from build123d import *

# Parameters (mm, degrees)
BOSS_EXTRUDE1_START = 20
BOSS_EXTRUDE1_DEPTH = 20
CIRPATTERN1_COUNT   = 9


with BuildPart() as part:
    # Sketch1 → Revolve1 (revolve)
    with BuildSketch(Plane.XY):
        Polygon((-50, 0), (-50, 100), (0, 100), (0, 420), (-30, 420), (-30, 465), (-10, 465), (10.490381057, 459.509618943), (30, 440), (30, 0), align=None)
    revolve(axis=Axis((30, 0, 0), (-1, 0, 0)))

    # Sketch2 → Boss-Extrude1 (add)
    with BuildSketch(Plane.ZY.offset(BOSS_EXTRUDE1_START)):
        with BuildLine():
            ThreePointArc((27.272727273, 96.209138584), (22.022759648, 99.799825551), (20, 105.830052443))
            Line((20, 105.830052443), (20, 408.900966005))
            ThreePointArc((20, 408.900966005), (23.192543543, 416.226164746), (30.731707317, 418.874160298))
            ThreePointArc((30.731707317, 418.874160298), (5.43490171, 419.964834056), (-19.881656805, 419.529164329))
            ThreePointArc((-19.881656805, 419.529164329), (-56.82924306, 416.1375219), (-93.333333333, 409.498338078))
            ThreePointArc((-93.333333333, 409.498338078), (-42.583426132, 397.902733094), (-20, 350.998575496))
            Line((-20, 350.998575496), (-20, 105.830052443))
            ThreePointArc((-20, 105.830052443), (-22.022759648, 99.799825551), (-27.272727273, 96.209138584))
            ThreePointArc((-27.272727273, 96.209138584), (0, 100), (27.272727273, 96.209138584))
        make_face()
    boss_extrude1 = extrude(amount=-BOSS_EXTRUDE1_DEPTH)

    # CirPattern1: Boss-Extrude1 ×9 about axis
    cirpattern1_axis = Axis((0, 0, 0), (1, 0, 0))
    for i in range(1, CIRPATTERN1_COUNT):
        add(boss_extrude1.rotate(cirpattern1_axis, i * 360 / CIRPATTERN1_COUNT))


solid = part.part
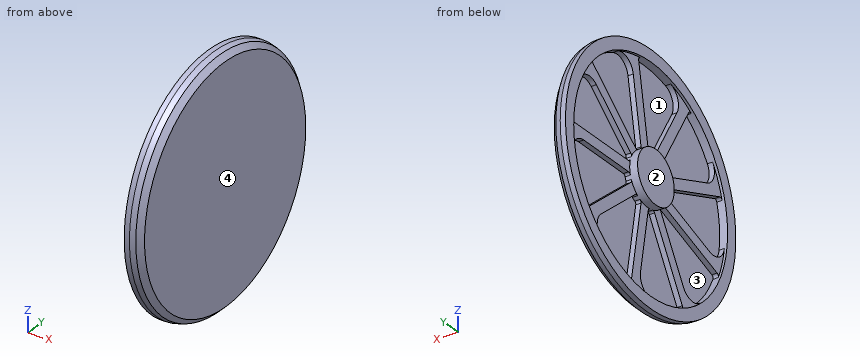
Source: CAD feature listing. Evaluate the final solid. Frame: model axes, mm. Face numbers are marked on the shaded views. A direction names the side the tool comes from. Coordinates: 2 decimals unless noted, no trailing zeros. Write each question's results on one line, items separated by ' | '. Start each with the question number.
1. Draft query along Z for the marked faces 1 and 2. Return one class per face: +Z half, -Z half, draft (parallel to the pull), parting line (faces both ways), or undercut.
2. Material intervals for L1, parallel to Z at x = -20.5, y = 0; L2, parallel to Y at x = -19, z = 0; L3, parallel to X at y = -207.5, z = -217, sorted ascending.
3. Pin query (flat end, axial travel): pin 1 (5 mm diameter, centred on x = -19.5, y = -231.5, fed in from +Z); pin 2 (8 mm diameter, centred on x = 6.5, y = 332.5, fed in from -Z); pin 3 (22 mm diameter, centred on x = -13, y = 208.5, fed in from +Z). Return the tip coordinate at first contact, or that it passes through.
4. Reachability of the marked faces 3 and 4 from +Z, -Z, +X, -X, +Y, -Y: full face, straight path, thin tool, end or side. Return the list, or none.
Solution:
1) face 1: undercut | face 2: draft
2) L1: -465 to -420, -100 to 100, 420 to 465 | L2: -465 to -420, -100 to 465 | L3: 0 to 30
3) pin 1: z = 404.7 | pin 2: z = -323.11 | pin 3: z = 420.97
4) face 3: -X | face 4: +Z, -Z, +X, +Y, -Y
